Could you check a few things on this model? Use its own coordinates, in mm. Give positions to 0.01 mm unless a question says otherwise; leave off trailing zeros. Write each loop counter-clockwise with the first axis right and the second up, starting at its lowest first coordinate (ties: lowest second). Pieces come first, ordered by that corner, then holes. Notation, with made-up numbers: (-13, 17) - (27, 17) arc R8 ccw to (27, 22) - close; hole circle Ø8 at (63, -6.5). An arc over 180 degrees is marked (long way). Write item = value, one per line.
from build123d import *

# Parameters (mm, degrees)
F0_W          = 177.8
F0_H          = 152.4
F1_DEPTH      = 6.35
F1_DEPTH_BACK = 6.35
F3_DEPTH      = 12.701


with BuildPart() as f1:
    # F0 (on Top) → F1 (new body, two sides)
    with BuildSketch(Plane.XY) as f1_sk:
        with Locations((12.7, 0)):
            Rectangle(F0_W, F0_H)
    extrude(amount=F1_DEPTH)
    extrude(f1_sk.sketch, amount=-F1_DEPTH_BACK)

    # F2 (on face) → F3 (cut, through all)
    with BuildSketch(Plane.XY.offset(6.35)):
        with BuildLine():
            ThreePointArc((-47.625, -2.2225), (-44.45, -5.3975), (-41.275, -2.2225))
            ThreePointArc((-41.275, -2.2225), (-44.45, 0.9525), (-47.625, -2.2225))
        make_face()
        with BuildLine():
            ThreePointArc((-6.35, -2.2225), (-9.525, 0.9525), (-12.7, -2.2225))
            ThreePointArc((-12.7, -2.2225), (-9.525, -5.3975), (-6.35, -2.2225))
        make_face()
        with BuildLine():
            ThreePointArc((-23.8125, -2.2225), (-26.9875, 0.9525), (-30.1625, -2.2225))
            ThreePointArc((-30.1625, -2.2225), (-26.9875, -5.3975), (-23.8125, -2.2225))
        make_face()
    extrude(amount=-F3_DEPTH, mode=Mode.SUBTRACT)


solid = f1.part
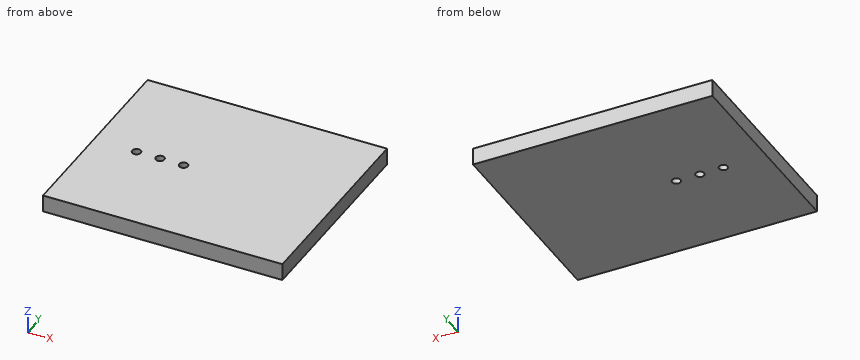
1. If we section it at A-A, the plane x = -44.45: Please give me the cut outline in (y, z), and give its area (3 significant figures).
Filled sheet:
outline = (-76.2, -6.35) - (-5.4, -6.35) - (-5.4, 6.35) - (-76.2, 6.35) - close; (0.95, -6.35) - (76.2, -6.35) - (76.2, 6.35) - (0.95, 6.35) - close
area = 1,850 mm2
2. For pin 1 (5.5 mm diameter, centred on x = -9.52, y = -2.22, fed in from +Z), with a flat end and sliding along its axis, tell me the tip position at first contact or that it passes through.
Filled sheet:
pin_1 = through
3. I need wall thicknesses on line 1 (X direction, y = -5, z = 5.25); line 2 (Y direction, x = -29, z = 2.75); line 3 (Y direction, x = -25, z = 2.25). Which ranges of each line are inside material? Lowest first, please.
Filled sheet:
line_1 = -76.2 to -45.99, -42.91 to -28.53, -25.45 to -11.06, -7.99 to 101.6
line_2 = -76.2 to -4.68, 0.23 to 76.2
line_3 = -76.2 to -4.7, 0.25 to 76.2
